Answer from the drawing. Dimensions are ordinates in mm from the lowest x, y and z of the part. Coordinates: 2 decimals unless noted, no trailing zeros. Write each loop counter-clockwise with the first axis right and the second up, starting at its lowest first coordinate (ties: lowest second). Pieces come first, ordered by that corner, then holes.
(1) Given pin 1 (2 mm diameter, centred on y = 11, z = 232.5, fed in from -X), flat-ended and moving along its own axis, determine where the tip first touches the part or whether it passes through.
(2) Section B-B on z = 777.5 is taken. Write down the section's boundary in (x, y), then the cut area to 3 significant figures.
(3) Section C-C on y = 9.5 is taken. Write down the section's boundary in (x, z), then the cut area to 3 significant figures.
(4) Find the intervals of material crossed by probe 1 along X at (y, z) = (34, 604.5); probe 2 along Z at (x, y) = (268, 13), in increasing order.
(5) Section A-A on x = 258.5 is taken. Write down the section's boundary in (y, z), then the cut area to 3 significant figures.
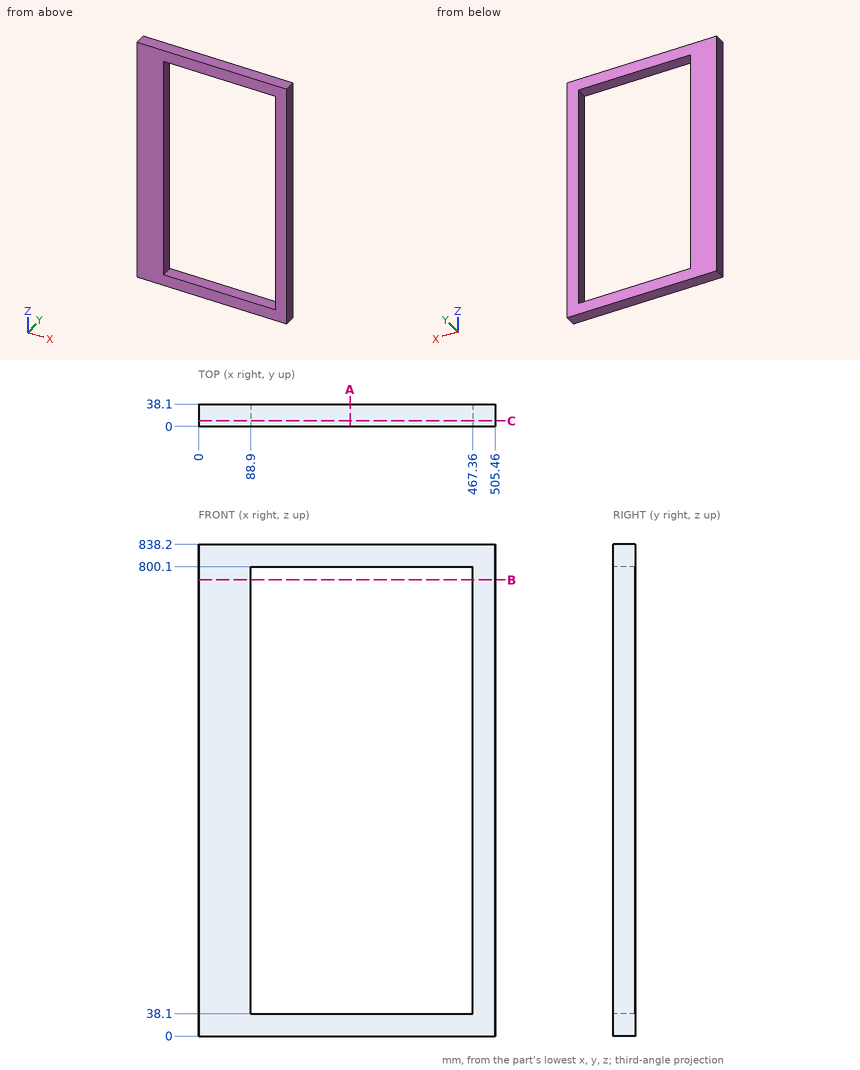
Response:
1. pin 1: stops at x = 0
2. outline: (0, 0) - (88.9, 0) - (88.9, 38.1) - (0, 38.1) - close; (467.36, 0) - (505.46, 0) - (505.46, 38.1) - (467.36, 38.1) - close
2. area: 4,840 mm2
3. outline: (0, 0) - (505.46, 0) - (505.46, 838.2) - (0, 838.2) - close; hole (88.9, 38.1) - (467.36, 38.1) - (467.36, 800.1) - (88.9, 800.1) - close
3. area: 135,000 mm2
4. probe 1: x = 0 to 88.9, 467.36 to 505.46
4. probe 2: z = 0 to 38.1, 800.1 to 838.2
5. outline: (0, 0) - (38.1, 0) - (38.1, 38.1) - (0, 38.1) - close; (0, 800.1) - (38.1, 800.1) - (38.1, 838.2) - (0, 838.2) - close
5. area: 2,900 mm2
